The listing builds one solid part. Answer for the finished solid, in the listing's coordinates (mm). Face numbers are marked on the shaded views. A direction names the side the tool comes from. Give positions to 0.01 mm unless a question says otherwise; leave off trailing zeros. Write each loop counter-clockwise with the first axis right and the second up, starting at its lowest first coordinate (ties: lowest second). Pieces come first, ordered by that corner, then holes. Notation, with made-up numbers: M -29,-11.75 L 5,-11.75 A19 cw 5,9.25 Z; hole C 74.5,81 d10. An arc over 180 degrees is marked long. Answer as a JSON object with one key per item and string values.
```python
from build123d import *

# Parameters (mm, degrees)
F0_W           = 7.4676
F0_H           = 9.652
F0_R           = 1
F1_DEPTH       = 5.08
F2_D           = 2
F2_CSINK_D     = 4
F2_CSINK_ANGLE = 90
F3_W           = 5.08
F3_H           = 5.658844
F3_R           = 1
F4_DEPTH       = 3.08102


with BuildPart() as f1:
    # F0 (on Front) → F1 (new body)
    with BuildSketch(Plane.XZ):
        Rectangle(F0_W, F0_H)
        with Locations((0, 0.6604)):
            Circle(F0_R, mode=Mode.SUBTRACT)
        with Locations((0, 0.6604)):
            Circle(F0_R)
    extrude(amount=-F1_DEPTH)

    # F2 (through all)
    with Locations(Plane.XZ):
        with Locations((0, 0.6604)):
            CounterSinkHole(F2_D / 2, F2_CSINK_D / 2, counter_sink_angle=F2_CSINK_ANGLE)

    # F3 (on face) → F4 (cut)
    with BuildSketch(Plane(origin=(0, 5.08, 0), x_dir=(-1, 0, 0), z_dir=(0, 1, 0))):
        with Locations((0, 0.6604)):
            Rectangle(F3_W, F3_H)
        with Locations((0, 0.6604)):
            Circle(F3_R, mode=Mode.SUBTRACT)
    extrude(amount=-F4_DEPTH, mode=Mode.SUBTRACT)


solid = f1.part
```
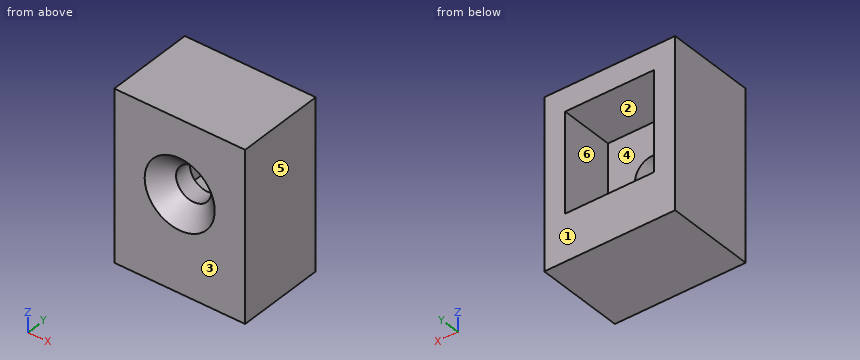
1. A cutting plane is placed at C-C, the plane z = 3. Give the vertices of the cut face in (x, y), plus the area to 3 significant figures.
Verdict:
{"outline": "M -3.73,0 L 3.73,0 L 3.73,5.08 L 2.54,5.08 L 2.54,2 L -2.54,2 L -2.54,5.08 L -3.73,5.08 Z", "area": "22.3 mm2"}
2. For the marked faces 1 and 2, determine the directions among +Z, -Z, +X, -X, +Y, -Y from which every point of the face is accessible in a straight line to the end or side of a thin tool.
Verdict:
{"face 1": "+Z, -Z, +X, -X, +Y", "face 2": "+Y"}
3. Consider line 1 along X through (y, z) = (4, -1); line 2 along Z through (x, y) = (0, 1.4); line 3 along Z through (x, y) = (2.5, 3.8). Determine where each line is inside the solid, lowest interval first.
Verdict:
{"line 1": "x = -3.73 to -2.54, 2.54 to 3.73", "line 2": "z = -4.83 to -0.34, 1.66 to 4.83", "line 3": "z = -4.83 to -2.17, 3.49 to 4.83"}
4. Flat-ended cylindrical pins translate along their axes: pin 1 (2.5 mm diameter, centred on x = 0, z = 0.66, fed in from -Y); pin 2 (3 mm diameter, centred on x = -1, z = 2, fed in from -Y). Find the tip coordinate at first contact, or state that the pin passes through.
Verdict:
{"pin 1": "stops at y = 0.75", "pin 2": "stops at y = 0"}
5. A cutting plane is placed at B-B, the plane y = 3.7. Give the vertices of the cut face in (x, z).
Verdict:
{"outline": "M -3.73,-4.83 L 3.73,-4.83 L 3.73,4.83 L -3.73,4.83 Z; hole M -2.54,-2.17 L 2.54,-2.17 L 2.54,3.49 L -2.54,3.49 Z"}
6. The mould has two halves that part along X. Classify the marked faces 3, 4, 5 and 6: released by +X, released by -X, zero draft, split by the parting line, or undercut.
Verdict:
{"face 3": "zero draft", "face 4": "undercut", "face 5": "released by +X", "face 6": "undercut"}
7. A cutting plane is placed at A-A, the plane x = 0. Give the vertices of the cut face in (y, z).
Verdict:
{"outline": "M 0,-4.83 L 5.08,-4.83 L 5.08,-2.17 L 2,-2.17 L 2,-0.34 L 1,-0.34 L 0,-1.34 Z; M 0,2.66 L 1,1.66 L 2,1.66 L 2,3.49 L 5.08,3.49 L 5.08,4.83 L 0,4.83 Z"}
